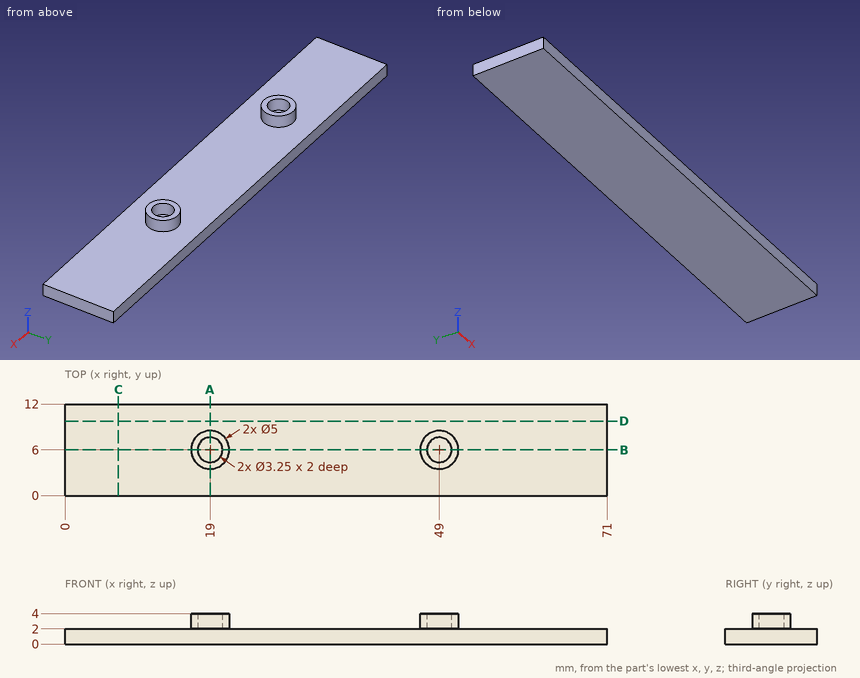
Geometry check sheet. Reference: drawing and pictorial views, mm from the part's lowest x, y, z. Give positions to 0.01 mm unless a question says otherwise; leave off trailing zeros. Write each loop counter-clockwise with the first axis right and the second up, starting at its lowest first coordinate (ties: lowest second). Pieces come first, ordered by that corner, then holes. Notation, with made-up numbers: M 36.5,21.5 L 57.5,21.5 A34 ccw 57.5,55.5 Z; hole C 56.25,65 d6. An arc over 180 degrees is marked long. Put each result on its own line as item: value. Start each with the question number.
1. Go/stop test with a flat-tipped pin: pin 1 Ø1 at (x, y) = (19, 7) entering from +Z. Record where the tip stops, or that it passes through.
2. Section check A-A (x = 19). Record the cut outline in (y, z) (3 decimals), and give its area (3 significant figures).
3. Section check B-B (y = 6). Record the cut outline in (x, z) (3 decimals).
4. Section check D-D (y = 9.75). Record the cut outline in (x, z).
5. Section check C-C (x = 7). Record the cut outline in (y, z).
6. Scan lines: line 1 along Y through (x, z) = (49, 3.5) (3 decimals); line 2 along Z through (x, y) = (37.5, 11.5); line 3 along X through (y, z) = (7, 3.3). Record each from-to range of solid material in increasing order. Write a range as [from, to].
Answer list:
1. pin 1: z = 2
2. outline: M 0,0 L 12,0 L 12,2 L 8.5,2 L 8.5,4 L 7.625,4 L 7.625,2 L 4.375,2 L 4.375,4 L 3.5,4 L 3.5,2 L 0,2 Z
2. area: 27.5 mm2
3. outline: M 0,0 L 71,0 L 71,2 L 51.5,2 L 51.5,4 L 50.625,4 L 50.625,2 L 47.375,2 L 47.375,4 L 46.5,4 L 46.5,2 L 21.5,2 L 21.5,4 L 20.625,4 L 20.625,2 L 17.375,2 L 17.375,4 L 16.5,4 L 16.5,2 L 0,2 Z
4. outline: M 0,0 L 71,0 L 71,2 L 0,2 Z
5. outline: M 0,0 L 12,0 L 12,2 L 0,2 Z
6. line 1: [3.5, 4.375], [7.625, 8.5]
6. line 2: [0, 2]
6. line 3: [16.71, 17.72], [20.28, 21.29], [46.71, 47.72], [50.28, 51.29]
